from build123d import *

# Parameters (mm, degrees)
BOSS_EXTRUDE1_DEPTH = 6.35
SKETCH2_R           = 1.7
CUT_EXTRUDE1_DEPTH  = 128.158650905
SKETCH3_W           = 101.6
SKETCH3_H           = 6.35
BOSS_EXTRUDE2_DEPTH = 50.8


with BuildPart() as part:
    # Sketch1 → Boss-Extrude1 (new body)
    with BuildSketch(Plane(origin=(0, 0, 0), x_dir=(1, 0, 0), z_dir=(0, 1, 0))):
        Polygon((15.24, 20.32), (15.24, 66.04), (60.96, 66.04), (60.96, 20.32), (65.96, 0), (76.2, 0), (76.2, 101.6), (0, 101.6), (0, 0), (10.24, 0), align=None)
    extrude(amount=BOSS_EXTRUDE1_DEPTH)

    # Sketch2 → Cut-Extrude1 (cut, through all)
    with BuildSketch(Plane(origin=(0, 6.35, 0), x_dir=(1, 0, 0), z_dir=(0, 1, 0))):
        with Locations(Location((5, 96.6, 0), (0, 0, 270))):
            Circle(SKETCH2_R)
        with Locations(Location((71.2, 96.6, 0), (0, 0, 90))):
            Circle(SKETCH2_R)
        with Locations(Location((71.2, 5, 0), (0, 0, 270))):
            Circle(SKETCH2_R)
        with Locations(Location((5, 5, 0), (0, 0, 90))):
            Circle(SKETCH2_R)
    extrude(amount=-CUT_EXTRUDE1_DEPTH, mode=Mode.SUBTRACT)


with BuildPart() as body_2:
    # Mirror1: mirrored copy
    add(part.part.mirror(Plane.ZY.offset(25.4)))


with BuildPart() as part_1:
    add(part.part)

    add(body_2.part)  # Boss-Extrude2 merges body 2
    # Sketch3 → Boss-Extrude2 (add)
    with BuildSketch(Plane(origin=(-50.8, 0, 0), x_dir=(0, 0, -1), z_dir=(1, 0, 0))):
        with Locations((50.8, 3.175)):
            Rectangle(SKETCH3_W, SKETCH3_H)
    extrude(amount=BOSS_EXTRUDE2_DEPTH)


solid = part_1.part
Source: CAD feature listing. Evaluate the final solid. Frame: model axes, mm. A direction names the side the tool comes from. Round coordinates to 2 decimals unless told otherwise and drop trailing zeros. Loops run counter-clockwise (first coordinate to the right, second up) from the corner with the lowest first, then second, coordinate; pieces in that order, holes last.
Q1. First-contact query: P1, Ø1.9, axis at x = -100, y = 2.5, coming from the +Z side. Flat tip, straight axial feed; report the tip coordinate or a pass-through.
Q2. Section C-C, the plane x = 40. Return loops of the section in (y, z), plus the area to 3 significant figures.
Q3. Ray query, line 1 (X direction, y = 2.75, z = -96.6); line 2 (X direction, y = 3.75, z = -33); line 3 (Z direction, x = 71.2, y = 3). Return the intervals inside material, ascending.
Q4. Section B-B, the plane z = -13.5. Return loops of the section in (x, y).
Q5. Access query for faces 4 (the face through (-27, 6.35, -61)), 5 (the face through (-63.5, 3.1, -10)). Directions: +Z, -Z, +X, -X, +Y, -Y. A direction counts if a zero-diameter tool reaches every point of the face in a straight line with its end or side. Return the directions, or none.
Q6. Section A-A, the plane z = -42. Return loops of the section in (x, y).
Q7. Mould query, pull axis X, two halves, no side actions, for faces 1 (the face through (-66.04, 3, -43)), 2 (the face through (-27, 3, -101.6)), 3 (the face through (-127, 3, -50)). Classes: pulls with the +X half, pulls with the -X half, needs draft (parallel to the pull), parting line crosses it, or undercut.
Solutions:
1. P1: stops at z = -66.04
2. outline: (0, -101.6) - (6.35, -101.6) - (6.35, -66.04) - (0, -66.04) - close
2. area: 226 mm2
3. line 1: x = -127 to -123.7, -120.3 to -57.5, -54.1 to 3.3, 6.7 to 69.5, 72.9 to 76.2
3. line 2: x = -127 to -111.76, -66.04 to 15.24, 60.96 to 76.2
3. line 3: z = -101.6 to -98.3, -94.9 to -6.7, -3.3 to 0
4. outline: (-127, 0) - (-113.44, 0) - (-113.44, 6.35) - (-127, 6.35) - close; (-64.36, 0) - (13.56, 0) - (13.56, 6.35) - (-64.36, 6.35) - close; (62.64, 0) - (76.2, 0) - (76.2, 6.35) - (62.64, 6.35) - close
5. face 4: +Z, -Z, +X, -X, +Y
5. face 5: +Z, +Y, -Y
6. outline: (-127, 0) - (-111.76, 0) - (-111.76, 6.35) - (-127, 6.35) - close; (-66.04, 0) - (15.24, 0) - (15.24, 6.35) - (-66.04, 6.35) - close; (60.96, 0) - (76.2, 0) - (76.2, 6.35) - (60.96, 6.35) - close
7. face 1: undercut
7. face 2: needs draft
7. face 3: pulls with the -X half
